The model under review builds one solid part; all positions refer to its coordinate system, in mm. A direction names the side the tool comes from. Give positions to 0.01 mm unless a question says otherwise; leave off trailing zeros. Loops run counter-clockwise (first coordinate to the right, second up) from the corner with the lowest first, then second, coordinate; pieces in that order, holes last. Notation, with made-up numbers: (48, 6.5) -> (99, 6.5) arc R25 cw to (99, 26.5) -> close; hole circle Ø1 at (52.5, 23). An arc over 180 degrees is marked (long way). Write each question's results on one line, items separated by ' | '. Start each with the question number.
Q1. Insertion check: pin 1 Ø0.7 at (x, z) = (-3.5, 18.5) entering from +Y; pin 2 Ø0.6 at (x, z) = (-5.5, 13) entering from -Y; pin 3 Ø3.5 at (y, z) = (4.92, 14.44) entering from -X. Each pin has a flat end and moves straight along its axis. Give the tip position at first contact, or say it passes through.
Q2. Wall thickness on L1, parallel to X at y = -1, z = 13.75; L2, parallel to Y at x = -1, z = 15; L3, parallel to X at y = 2.25, z = 13.25: over which ranges is each line inside the solid? List them lowest first. Write a range as [from, to].
Q3. We need section C-C (x = -6.75). Write out the cut boundary in (y, z) (3 decimals), plus the area to 3 significant figures.
Q4. We need section D-D (z = 12). Write out the cut boundary in (x, y), plus the area to 3 significant figures.
Q5. We need section A-A (y = 5.5). Write out the cut boundary in (x, z).
Q6. We need section B-B (z = 15.75). Write out the cut boundary in (x, y).
Q7. Machinability: for faces 4 (the face through (-4, -3, 19.313)), 5 (the face through (-0.81, 6.32, 11.98)), 6 (the face through (-4, 1.1, 19)), 7 (the face through (-4, -3, 12.413)), which of the approach directions +Z, -Z, +X, -X, +Y, -Y give a long, thin tool a straight path to every point of the face, cutting with its end or side? Answer none if there is none.
Q8. Mouldability with a two-part tool opening along Z and no side actions: class faces 1 (the face through (0.369, -1, 15)), 2 (the face through (-4, 1, 10.913)), 3 (the face through (-1, 7.75, 14)) as released by +Z, released by -Z, zero draft, split by the parting line, or undercut.
from build123d import *

# Parameters (mm, degrees)
SKETCH007_R     = 1.85
PAD003_DEPTH    = 9
POCKET003_DEPTH = 8
POCKET004_DEPTH = 2.4


with BuildPart() as part:
    # Sketch007 (on Face1 of ReferencePolarPattern) → Pad003 (new body)
    with BuildSketch(Plane.YZ.offset(-13.630613)):
        Polygon((-7.3, 19.312846), (1.1, 19.312846), (1.1, 17.862846), (8.35, 17.862846), (8.35, 10.912846), (-7.3, 10.912846), align=None)
        with Locations((4.925, 14.437846)):
            Circle(SKETCH007_R, mode=Mode.SUBTRACT)
    extrude(amount=PAD003_DEPTH)

    # Sketch008 (on Face6 of Pad003) → Pocket003 (cut)
    with BuildSketch(Plane(origin=(0, -7.3, 0), x_dir=(0, 0, -1), z_dir=(0, -1, 0))):
        with BuildLine():
            ThreePointArc((-14.012846, -13.130613), (-13.512846, -12.630613), (-14.012846, -12.130613))
            ThreePointArc((-14.012846, -11.130613), (-14.512846, -11.630613), (-14.012846, -12.130613))
            ThreePointArc((-14.012846, -11.130613), (-13.512846, -10.630613), (-14.012846, -10.130613))
            ThreePointArc((-14.012846, -9.130613), (-14.512846, -9.630613), (-14.012846, -10.130613))
            ThreePointArc((-14.012846, -9.130613), (-13.512846, -8.630613), (-14.012846, -8.130613))
            ThreePointArc((-14.012846, -7.130613), (-14.512846, -7.630613), (-14.012846, -8.130613))
            ThreePointArc((-14.012846, -7.130613), (-13.512846, -6.630613), (-14.012846, -6.130613))
            ThreePointArc((-14.012846, -5.130613), (-14.512846, -5.630613), (-14.012846, -6.130613))
            ThreePointArc((-14.012846, -5.130613), (-13.6592926094, -4.9841663906), (-13.512846, -4.630613))
            Line((-12.412846, -4.630613), (-13.512846, -4.630613))
            Line((-12.412846, -13.630613), (-12.412846, -4.630613))
            Line((-14.512846, -13.630613), (-12.412846, -13.630613))
            ThreePointArc((-14.012846, -13.130613), (-14.3663993906, -13.2770596094), (-14.512846, -13.630613))
        make_face()
    extrude(amount=-POCKET003_DEPTH, mode=Mode.SUBTRACT)

    # Sketch009 (on Face5 of Pocket003) → Pocket004 (cut)
    with BuildSketch(Plane.YZ.offset(-4.630613)):
        Polygon((7.75, 12.8068314895), (7.75, 16.0688605105), (4.925, 17.6998750209), (2.1, 16.0688605105), (2.1, 12.8068314895), (4.925, 11.1758169791), align=None)
    extrude(amount=-POCKET004_DEPTH, mode=Mode.SUBTRACT)


with BuildPart() as part_1:
    # Body001 placement: moved
    add(part.part.moved(Location((5, 0, 0))))


solid = part_1.part
Output:
1) pin 1: y = 1.1 | pin 2: y = 0.7 | pin 3: through
2) L1: [-8.06, -7.21], [-6.06, -5.21], [-4.06, -3.21], [-2.06, -1.21], [-0.06, 0.37] | L2: [-7.3, 2.1], [7.75, 8.35] | L3: [-8.63, -2.03]
3) outline: (-7.3, 10.913) -> (8.35, 10.913) -> (8.35, 17.863) -> (1.1, 17.863) -> (1.1, 19.313) -> (-7.3, 19.313) -> (-7.3, 14.498) -> (0.7, 14.498) -> (0.7, 12.413) -> (-7.3, 12.413) -> close; hole circle Ø3.7 at (4.925, 14.438) | area: 93.5 mm2
4) outline: (-8.63, -7.3) -> (0.37, -7.3) -> (0.37, 3.5) -> (-2.03, 3.5) -> (-2.03, 6.35) -> (0.37, 6.35) -> (0.37, 8.35) -> (-8.63, 8.35) -> close | area: 134 mm2
5) outline: (-8.63, 10.91) -> (0.37, 10.91) -> (0.37, 11.51) -> (-2.03, 11.51) -> (-2.03, 12.68) -> (-8.63, 12.68) -> close; (-8.63, 16.2) -> (-2.03, 16.2) -> (-2.03, 17.37) -> (0.37, 17.37) -> (0.37, 17.86) -> (-8.63, 17.86) -> close
6) outline: (-8.63, -7.3) -> (0.37, -7.3) -> (0.37, 2.1) -> (-2.03, 2.1) -> (-2.03, 3.62) -> (-8.63, 3.62) -> close; (-8.63, 6.23) -> (-2.03, 6.23) -> (-2.03, 7.75) -> (0.37, 7.75) -> (0.37, 8.35) -> (-8.63, 8.35) -> close
7) face 4: +Z, +X, -X, +Y, -Y | face 5: +X | face 6: +Z, +X, -X, +Y | face 7: +X, -X, -Y
8) face 1: zero draft | face 2: released by -Z | face 3: undercut
